```python
from build123d import *

# Parameters (mm, degrees)
PAD_DEPTH = 15.8


with BuildPart() as part:
    # Sketch → Pad (new body)
    with BuildSketch(Plane.XY):
        with BuildLine():
            Line((-15, 50), (15, 50))
            ThreePointArc((40, 48), (27.516552, 49.206897), (15, 50))
            Line((40, 51.5), (40, 48))
            Line((-40, 51.5), (40, 51.5))
            Line((-40, 48), (-40, 51.5))
            ThreePointArc((-15, 50), (-27.516552, 49.206897), (-40, 48))
        make_face()
    extrude(amount=PAD_DEPTH)


solid = part.part
```
Geometry check sheet. Reference: the model listing, model coordinates, mm. A direction names the side the tool comes from. Coordinates: 2 decimals unless noted, no trailing zeros. Order: outer loops, then holes, each group sorted by start corner. A loop starts at its lowest first (then second) coordinate and runs counter-clockwise, first axis right, second up. Notation, with made-up numbers: (19.5, -4.5) - (49.5, -4.5) arc R22 cw to (49.5, 29.5) - close; hole circle Ø10 at (76, 2.25). An arc over 180 degrees is marked (long way). Answer as a JSON object with one key per item and string values. Group by question number.
Item 1: Sectioned sample at D-D, the plane x = 33. Record the cut outline in (y, z).
Item 2: Sectioned sample at B-B, the plane z = 2. Record the cut outline in (x, y), and give its area (3 significant figures).
Item 3: Sectioned sample at C-C, the plane x = -13. Record the cut outline in (y, z), and give its area (3 significant figures).
Item 4: Depth check by flat-ended pin: pin 1 Ø2 at (x, y) = (15.5, 50) entering from -Z; pin 2 Ø4 at (x, z) = (21, 12) entering from -Y. Enter the tip coordinate at first touch or a pass-through.
Item 5: Scan lines: probe 1 along Y at (x, z) = (-8.5, 4.75); probe 2 along Y at (x, z) = (-26, 11.75). Record each from-to range of solid material in increasing order.
Item 6: Tool access check on faces 1 (the face through (27.692, 49.193, 7.789)), 2 (the face through (-1, 51.5, 8)). Record the directions out of +Z, -Z, +X, -X, +Y, -Y that give a thin tool (end or side, any length) a straight path to the whole face; none if there is none.
Resolved:
{
 "1": {"outline": "(48.73, 0) - (51.5, 0) - (51.5, 15.8) - (48.73, 15.8) - close"},
 "2": {"outline": "(-40, 48) arc R378.91 cw to (-15, 50) - (15, 50) arc R378.91 cw to (40, 48) - (40, 51.5) - (-40, 51.5) - close", "area": "163 mm^2"},
 "3": {"outline": "(50, 0) - (51.5, 0) - (51.5, 15.8) - (50, 15.8) - close", "area": "23.7 mm^2"},
 "4": {"pin 1": "z = 0", "pin 2": "y = 49.54"},
 "5": {"probe 1": "50 to 51.5", "probe 2": "49.33 to 51.5"},
 "6": {"face 1": "+Z, -Z, -Y", "face 2": "+Z, -Z, +X, -X, +Y"}
}
